Autodesk Inventor part; units mm, degrees
ref_plane "YZ Plane" through (0, 0, 0) normal (1, 0, 0) x (0, 1, 0)
ref_plane "XZ Plane" through (0, 0, 0) normal (0, 1, 0) x (-1, 0, 0)
ref_plane "XY Plane" through (0, 0, 0) normal (0, 0, 1) x (1, 0, 0)
sketch "Skizze1" plane through (0, 0, 0) normal (0, 0, 1) x (1, 0, 0)
  line L0 (-56, 0) -> (336, 0)
  line L1 (0, -23) -> (0, 138)
  line L2 (0, 0) -> (280, 0)
  line L3 (280, 0) -> (280, 115)
  line L4 (280, 115) -> (0, 115)
  line L5 (0, 115) -> (0, 0)
  line L6 (5, 110) -> (275, 110)
  line L7 (275, 110) -> (275, 5)
  line L8 (275, 5) -> (5, 5)
  line L9 (5, 5) -> (5, 110)
  point P0 (0, 115)
  dimension "d0" = 280
  dimension "d1" = 115
  dimension "d2" = 5
  dimension "d3" = 5
  dimension "d4" = 5
  dimension "d5" = 5
extrude "Extrusion1" add sketch "Skizze1" along normal blind 50
sketch "Skizze2" plane through (0, 0, 50) normal (0, 0, 1) x (1, 0, 0)
  point P0 (0, 0)
sketch "Skizze3" plane through (0, 0, 50) normal (0, 0, 1) x (1, 0, 0)
  line L0 (0, 115) -> (0, 0)
  line L1 (0, 0) -> (280, 0)
  line L2 (0, 115) -> (280, 115)
  line L3 (280, 115) -> (280, 0)
  line L4 (280, 0) -> (0, 0)
  line L5 (0, 0) -> (0, 115)
  line L6 (280, 115) -> (0, 115)
  line L7 (280, 0) -> (0, 0)
  line L8 (0, 0) -> (0, 115)
  line L9 (0, 115) -> (280, 115)
  line L10 (280, 115) -> (280, 0)
extrude "Extrusion2" add sketch "Skizze3" along normal blind 30
fillet "Rundung1" radius 52 4 edges at (140, 115, 80) (140, 0, 80) (0, 57.5, 80) (280, 57.5, 80)
sketch "Skizze5" plane through (0, 0, 0) normal (0, 0, -1) x (-1, 0, 0)
  line L0 (-5, 110) -> (-275, 110)
  line L1 (-182.5, 110) -> (-182.5, 5)
  line L2 (-275, 5) -> (-5, 5)
  line L3 (-92.5, 110) -> (-92.5, 5)
  line L4 (-275, 110) -> (-275, 5)
  line L5 (-177.5, 110) -> (-177.5, 5)
  line L6 (-87.5, 110) -> (-87.5, 5)
  point P0 (0, 0)
  dimension "d11" = 92.5
  dimension "d12" = 182.5
  dimension "d13" = 5
  dimension "d14" = 5
extrude "Extrusion3" add sketch "Skizze5" against normal blind 50 contours L6 L2 L3 L0 | L5 L2 L1 L0
sketch "Skizze6" plane through (0, 0, 80) normal (0, 0, 1) x (1, 0, 0)
  line L0 (52, 52) -> (52, 63)
  line L1 (228, 63) -> (228, 52)
  line L2 (177.5, 110) -> (177.5, 5)
  line L3 (52, 63) -> (228, 63)
  point P0 (0, 0)
  point P1 (67, 57)
  point P2 (136, 57)
  point P3 (213, 57)
  dimension "d17" = 15
  dimension "d18" = 15
  dimension "d19" = 41.5
  dimension "d20" = 6
  dimension "d21" = 6
  dimension "d22" = 6
hole "Bohrung1" at (67, 57, 80) at (136, 57, 80) at (213, 57, 80) direction (0, 0, -1) diameter 4 end through all
sketch "Skizze8" plane through (0, 0, 50) normal (0, 0, -1) x (-1, 0, 0)
  line L0 (-52, 95) -> (-228, 95)
  line L1 (-228, 95) -> (-228, 20)
  line L2 (-228, 20) -> (-52, 20)
  line L3 (-52, 20) -> (-52, 95)
  line L4 (-228, 63) -> (-228, 52)
  line L5 (-52, 52) -> (-52, 63)
  line L6 (-92.5, 110) -> (-177.5, 110)
  line L7 (-177.5, 5) -> (-92.5, 5)
  point P0 (0, 0)
  dimension "d30" = 0
  dimension "d31" = 0
  dimension "d32" = 15
  dimension "d33" = 15
extrude "Extrusion4" cut sketch "Skizze8" against normal blind 19
properties part number "DeckelKoch" material "Polyaryletherketon-Kunststoff"
Work out the finished part from the listing and answer in its coordinate system (mm). A direction names the side the tool comes from. Round coordinates to 2 decimals unless told otherwise and drop trailing zeros. Write each loop counter-clockwise with the first axis right and the second up, starting at its lowest first coordinate (ties: lowest second). Pieces come first, ordered by that corner, then holes. Notation, with made-up numbers: (72.5, -3.5) - (116.5, -3.5) arc R23 ccw to (116.5, 22.5) - close; hole circle Ø10 at (-28, -4). An arc over 180 degrees is marked (long way). Return JSON: item names as keys, results as strings. Group by question number.
Q1. The mould has two halves that part along Z. Classify faces 1 (the flat face through (37, 58, 50)), 2 (the flat face through (177.5, 58, 25)), 3 (the flat face through (90, 58, 50)): released by +Z, released by -Z, zero draft, split by the parting line, or undercut.
Q2. The part is cut by section A-A on x = 156. Write down the section's boundary in (y, z).
Q3. For faces 4 (the flat face through (138, 0, 14)), 5 (the flat face through (228, 110, 25)), determine the directions among +Z, -Z, +X, -X, +Y, -Y from which every point of the face is accessible in a straight line to the end or side of a thin tool.
Q4. Find the intervals of material crossed by L1, parallel to X at y = 5.5, z = 26.5; L2, parallel to X at y = 57, z = 73; L3, parallel to Y at x = 167.5, z = 6.5, in increasing order.
Q5. The part is cut by section B-B on z = 23. Write down the section's boundary in (x, y).
Q6. The part is cut by section C-C on y = 48. Write down the section's boundary in (x, z).
Q7. The part is cut by section D-D on x = 32. Write down the section's boundary in (y, z).
Q8. Each of these flat-tipped pins is pushed along its axis until it touches: pin 1 Ø1.5 at (x, y) = (129, 28.5) entering from -Z; pin 2 Ø5 at (y, z) = (85.5, 48) entering from -X; pin 3 Ø12 at (x, y) = (112, 83.5) entering from +Z. Where does it stop, or does it pass through?
Solved:
{
 "1": {"face 1": "released by -Z", "face 2": "zero draft", "face 3": "undercut"},
 "2": {"outline": "(0, 0) - (5, 0) - (5, 50) - (20, 50) - (20, 68.99) arc R52 ccw to (0, 28) - close; (20.02, 69) - (94.98, 69) arc R52 ccw to (63, 80) - (52, 80) arc R52 ccw to start; (95, 50) - (110, 50) - (110, 0) - (115, 0) - (115, 28) arc R52 ccw to (95, 68.99) - close"},
 "3": {"face 4": "+Z, -Z, +X, -X, -Y", "face 5": "-Z"},
 "4": {"L1": "0 to 5, 87.5 to 92.5, 177.5 to 182.5, 275 to 280", "L2": "25.94 to 65, 69 to 134, 138 to 211, 215 to 254.06", "L3": "0 to 5, 110 to 115"},
 "5": {"outline": "(0, 0) - (280, 0) - (280, 115) - (0, 115) - close; hole (5, 5) - (87.5, 5) - (87.5, 110) - (5, 110) - close; hole (92.5, 5) - (177.5, 5) - (177.5, 110) - (92.5, 110) - close; hole (182.5, 5) - (275, 5) - (275, 110) - (182.5, 110) - close"},
 "6": {"outline": "(0, 0) - (5, 0) - (5, 50) - (52, 50) - (52, 69) - (228, 69) - (228, 50) - (275, 50) - (275, 0) - (280, 0) - (280, 28) arc R52 ccw to (232, 79.85) - (48, 79.85) arc R52 ccw to (0, 28) - close; (87.5, 0) - (92.5, 0) - (92.5, 50) - (87.5, 50) - close; (177.5, 0) - (182.5, 0) - (182.5, 50) - (177.5, 50) - close"},
 "7": {"outline": "(0, 0) - (5, 0) - (5, 50) - (110, 50) - (110, 0) - (115, 0) - (115, 28) arc R52 ccw to (83, 76) - (32, 76) arc R52 ccw to (0, 28) - close"},
 "8": {"pin 1": "z = 69", "pin 2": "x = 3.03", "pin 3": "z = 77.94"}
}
